Could you check a few things on this model? Use its own coordinates, in mm. A direction names the side the tool comes from. Give positions to 0.01 mm unless a question says otherwise; leave off trailing zeros. Write each loop counter-clockwise with the first axis right and the second up, starting at its lowest first coordinate (ties: lowest second). Pieces come first, ordered by that corner, then holes. Notation, with made-up numbers: M 3.5,-28.75 L 42.5,-28.75 A24 cw 42.5,-13.75 Z; hole C -8.5,5 d2. An arc over 180 degrees is marked long. One line per item, written item: value.
Autodesk Inventor part; units mm, degrees
ref_plane "Work Plane1" through (0, 0, 0) normal (1, 0, 0) x (0, 1, 0)
ref_plane "XZ Plane" through (0, 0, 0) normal (0, 1, 0) x (-1, 0, 0)
ref_plane "XY Plane" through (0, 0, 0) normal (0, 0, 1) x (1, 0, 0)
sketch "Sketch1" plane through (0, 0, 0) normal (0, 1, 0) x (-1, 0, 0)
  line L0 (-3.25, 5) -> (-3.25, 0)
  line L1 (-3.25, 0) -> (3.25, 0)
  line L2 (3.25, 0) -> (3.25, 5)
  line L3 (2, 0) -> (-2, 0)
  line L4 (3, -43) -> (3, -78)
  line L5 (-3, -78) -> (-3, -43)
  line L6 (2, -118) -> (-2, -118)
  circle A0 centre (0, 5) radius 1.75
  arc A1 (3.25, 5) -> (-3.25, 5) centre (0, 5) ccw
  line L7 (2, 0) -> (3, -43)
  line L8 (-3, -43) -> (-2, 0)
  line L9 (3, -78) -> (2, -118)
  line L10 (-2, -118) -> (-3, -78)
  point P0 (0, 0)
  point P1 (0, 0)
  point P2 (0, 0)
  point P3 (0, -43)
  point P4 (0, -78)
  dimension "d0" = 6.5
  dimension "d1" = 5
  dimension "d2" = 6
  dimension "d3" = 4
  dimension "d4" = 3.5
  dimension "d5" = 90
  dimension "d6" = 91.332
  dimension "d7" = 88.568
  dimension "d8" = 91.332
  dimension "d9" = 88.568
  dimension "d10" = 118
  dimension "d11" = 0.25
  dimension "d12" = 6.25
  dimension "d13" = 1.9995
  dimension "d14" = 43
  dimension "d15" = 3.25
  dimension "d16" = 78
  dimension "d17" = 3.25
  dimension "d18" = 0
  dimension "d19" = 3.25
extrude "Extrusion1" add sketch "Sketch1" along normal blind 5
sketch "Sketch2" plane through (0, 5, 0) normal (0, 1, 0) x (1, 0, 0)
  circle A0 centre (0, 45) radius 1.25
  circle A1 centre (0, 71) radius 1.75
  circle A2 centre (0, -5) radius 1.75 construction
  circle A3 centre (0, -5) radius 1.75 construction
  point P0 (0, 0)
  point P1 (0, 0)
  dimension "d22" = 2.5
  dimension "d23" = 3.5
  dimension "d25" = 3.5
  dimension "d26" = 50
  dimension "d116" = 45
  dimension "d117" = 0
  dimension "d118" = 76
extrude "Extrusion2" cut sketch "Sketch2" against normal through all
sketch "Sketch6" plane through (2, 0, -118) normal (0, 0, -1) x (-1, 0, 0)
  line L0 (0, 5) -> (4, 5)
  line L1 (0.75, 5) -> (3.25, 5)
  line L2 (2, 5) -> (-2, 5)
  line L3 (2, 5) -> (6, 5)
  line L4 (6, 5) -> (6, 0)
  line L5 (6, 0) -> (-2, 0)
  line L6 (5.25, 0) -> (-1.25, 0)
  line L7 (-2, 0) -> (-2, 5)
  dimension "d43" = 4
  dimension "d44" = 4
  dimension "d45" = 5
  dimension "d46" = 8
extrude "Extrusion5" add sketch "Sketch6" along normal blind 5
ref_plane "Work Plane1" through (0, 0, 0) normal (1, 0, 0) x (0, 1, 0)
sketch "Sketch11" plane through (0, 0, 0) normal (1, 0, 0) x (0, 1, 0)
  line L0 (4.51, -121.065) -> (4.51, -116.065) construction
  line L1 (2.01, -122.9844) -> (4.01, -122.9844)
  line L2 (4.01, -122.9844) -> (5.26, -146.065)
  line L3 (5.26, -146.065) -> (2.01, -146.065)
  line L4 (2.01, -146.065) -> (2.01, -122.9844)
  line L5 (0, -118) -> (5, -118)
  line L6 (5, -43.75) -> (5, -46.25)
  line L7 (5, -69.25) -> (5, -72.75)
  line L8 (5, 6.75) -> (5, 3.25)
  line L9 (5, 5) -> (5, 5)
  line L10 (5, 5) -> (5, 0)
  line L11 (5, 0) -> (5, -43)
  line L12 (5, -43) -> (5, -78)
  line L13 (5, -78) -> (5, -118)
  line L14 (5, -118) -> (5, -123)
  line L15 (5, -118) -> (5, -123)
  line L16 (5, -118) -> (5, -78)
  line L17 (5, -78) -> (5, -43)
  line L18 (5, -43) -> (5, 0)
  line L19 (5, 0) -> (5, 5)
  line L20 (0.51, -143.3532) -> (0.51, -134.9626)
  line L21 (4.635, -134.5247) -> (4.635, -134.5247)
  line L22 (7.1466, -143.3532) -> (7.1466, -134.9626)
  point P0 (0, 0)
  point P1 (0, 0)
  dimension "d67" = 2
  dimension "d68" = 3.25
  dimension "d72" = 2.6467
  dimension "d73" = 30
  dimension "d76" = 2.6467
  dimension "d78" = 1.5
  dimension "d80" = 177.138
  dimension "d81" = 6.6366
  dimension "d82" = 3.1
  dimension "d107" = 0.49
  dimension "d109" = 16.9626
  dimension "d110" = 25.3532
  dimension "d111" = 3.065
  dimension "d112" = 16.9626
  dimension "d113" = 25.3532
  dimension "d114" = 7.1466
revolve "Revolution2" add sketch "Sketch11" angle 360 about axis through (0, 2.01, -146.065) along (0, 0, 1)
fillet "Fillet1" radius 3 1 edges at (0, -1.24, -146.065)
properties part number "reverse gear rever lever"
1) Please list where these lines run through material, in increasing order: L1, parallel to Z at x = 0, y = 2.4; L2, parallel to Z at x = 0, y = 2.15; L3, parallel to X at y = 1.75, z = -71. Write a range as from..to.
Outcome:
L1: z = -146.05..-72.75, -69.25..-46.25, -43.75..3.25, 6.75..8.25
L2: z = -146.06..-72.75, -69.25..-46.25, -43.75..3.25, 6.75..8.25
L3: x = -3..-1.75, 1.75..3
2) If we section it at B-B, the plane z = -71: Write out the boundary of the cut face in (x, y), then the cut area to 3 significant figures.
Outcome:
outline: M -3,0 L -1.75,0 L -1.75,5 L -3,5 Z; M 1.75,0 L 3,0 L 3,5 L 1.75,5 Z
area: 12.5 mm^2
3) I'm going to push flat-ended pins straight in: pin 1 (2 mm diameter, centred on x = 0, z = -45, fed in from -Y); pin 2 (1 mm diameter, centred on x = 0, z = -48.5, fed in from +Y); pin 3 (2.5 mm diameter, centred on y = 3, z = 2, fed in from -X); pin 4 (2.5 mm diameter, centred on y = 3, z = -68, fed in from +X). Where does each tip first touch, or does it pass through?
Outcome:
pin 1: passes through
pin 2: stops at y = 5
pin 3: stops at x = -3.25
pin 4: stops at x = 3
4) If we section it at C-C, the plane z = -108: Write out the boundary of the cut face in (x, y).
Outcome:
outline: M -2.25,0 L 2.25,0 L 2.25,5 L -2.25,5 Z
5) On a 3-axis mill with a long thin cutter (end or side, diameter ignored), from which of +Z, -Z, +X, -X, +Y, -Y can I reach the whole of each face in a straight line? I mean faces 1 (the face through (-3, 2, -60)), 2 (the face through (-2.26, 3.185, -133.091)), 3 (the face through (3.25, 2, 3)), 4 (the face through (3, 2, -61)). Say none if no direction works.
Outcome:
face 1: -X, +Y, -Y
face 2: none
face 3: +Z, +X, +Y, -Y
face 4: +X, +Y, -Y
6) If we section it at A-A, the plane z = -45: Write out the boundary of the cut face in (x, y), then the cut area to 3 significant figures.
Outcome:
outline: M -3,0 L -1.25,0 L -1.25,5 L -3,5 Z; M 1.25,0 L 3,0 L 3,5 L 1.25,5 Z
area: 17.5 mm^2
7) We'd pull the mould along Z, two halves only. Please class faces 5 (the face through (0.1, 4.2, -123)), 6 (the face through (0.07, 2.46, 8.25)), 7 (the face through (0, 0, -56)): pulls with the +Z half, pulls with the -Z half, needs draft (parallel to the pull), parting line crosses it, or undercut.
Outcome:
face 5: undercut
face 6: pulls with the +Z half
face 7: needs draft
